Autodesk Inventor part; units mm, degrees
ref_plane "YZ Plane" through (0, 0, 0) normal (1, 0, 0) x (0, 1, 0)
ref_plane "XZ Plane" through (0, 0, 0) normal (0, 1, 0) x (-1, 0, 0)
ref_plane "XY Plane" through (0, 0, 0) normal (0, 0, 1) x (1, 0, 0)
sketch "Sketch1" plane through (0, 0, 0) normal (0, 0, 1) x (1, 0, 0)
  line L0 (0, 0) -> (44.45, 0)
  line L1 (44.45, 0) -> (44.45, 3.302)
  line L2 (44.45, 3.302) -> (3.302, 3.302)
  line L3 (0, 31.75) -> (0, 0)
  line L4 (3.302, 3.302) -> (3.302, 31.75)
  line L5 (3.302, 31.75) -> (0, 31.75)
  line L6 (0, 31.75) -> (0, 0)
  point P0 (0, 3.302)
  dimension "d1" = 3.302
  dimension "d2" = 3.302
  dimension "d50" = 44.45
  dimension "d57" = 31.75
extrude "Extrusion1" add sketch "Sketch1" along normal blind 50.8
sketch "Sketch3" plane through (0, 0, 0) normal (-1, 0, 0) x (0, 0, 1)
  line L0 (0, 0) -> (50.8, 0) construction
  line L1 (0, 0) -> (12.7, 0) construction
  line L2 (12.7, 0) -> (25.4, 0) construction
  line L3 (25.4, 0) -> (38.1, 0) construction
  line L4 (38.1, 0) -> (38.1, 12.7) construction
  line L5 (38.1, 12.7) -> (38.1, 25.4) construction
  line L6 (25.4, 0) -> (25.4, 12.7) construction
  line L7 (25.4, 12.7) -> (25.4, 25.4) construction
  line L8 (12.7, 0) -> (12.7, 12.7) construction
  line L9 (12.7, 12.7) -> (12.7, 25.4) construction
  circle A0 centre (12.7, 25.4) radius 2.5797
  circle A1 centre (25.4, 25.4) radius 2.5797
  circle A2 centre (38.1, 25.4) radius 2.5797
  circle A3 centre (38.1, 12.7) radius 2.5797
  circle A4 centre (25.4, 12.7) radius 2.5797
  circle A5 centre (12.7, 12.7) radius 2.5797
  dimension "d9" = 12.7
  dimension "d10" = 12.7
  dimension "d11" = 12.7
  dimension "d12" = 12.7
  dimension "d13" = 12.7
  dimension "d14" = 12.7
  dimension "d15" = 12.7
  dimension "d16" = 12.7
  dimension "d17" = 12.7
  dimension "d18" = 5.1594
  dimension "d19" = 5.1594
  dimension "d20" = 5.1594
  dimension "d21" = 5.1594
  dimension "d22" = 5.1594
  dimension "d23" = 5.1594
extrude "Extrusion3" cut sketch "Sketch3" against normal blind 50.8
sketch "Sketch4" plane through (0, 0, 0) normal (0, -1, 0) x (1, 0, 0)
  line L0 (44.45, 0) -> (44.45, 50.8) construction
  line L1 (44.45, 50.8) -> (44.45, 38.1) construction
  line L2 (50.8, 38.1) -> (44.45, 38.1) construction
  line L3 (44.45, 38.1) -> (31.75, 38.1) construction
  line L4 (31.75, 38.1) -> (19.05, 38.1) construction
  line L5 (44.45, 0) -> (44.45, 13.462) construction
  circle A0 centre (31.75, 38.1) radius 2.5797
  circle A1 centre (19.05, 38.1) radius 2.5797
  line L6 (50.8, 12.7) -> (44.45, 12.7) construction
  line L7 (44.45, 12.7) -> (31.75, 12.7) construction
  line L8 (31.75, 12.7) -> (19.05, 12.7) construction
  line L9 (19.05, 12.7) -> (6.35, 12.7) construction
  circle A2 centre (31.75, 12.7) radius 2.5797
  circle A3 centre (19.05, 12.7) radius 2.5797
  line L10 (44.45, 13.462) -> (38.1, 13.462) construction
  line L11 (44.45, 12.7) -> (44.45, 17.4414) construction
  line L12 (19.05, 38.1) -> (6.35, 38.1) construction
  point P0 (0, 0)
  dimension "d26" = 12.7
  dimension "d27" = 6.35
  dimension "d28" = 12.7
  dimension "d29" = 12.7
  dimension "d31" = 13.462
  dimension "d33" = 5.1594
  dimension "d34" = 5.1594
  dimension "d37" = 6.35
  dimension "d38" = 12.7
  dimension "d39" = 12.7
  dimension "d40" = 12.7
  dimension "d42" = 5.1594
  dimension "d43" = 5.1594
  dimension "d53" = 12.7
extrude "Extrusion7" cut sketch "Sketch4" against normal blind 25.4
properties part number "2in bracket"
The listing builds one solid part. Answer for the finished solid, in the listing's coordinates (mm). A direction names the side the tool comes from. Give positions to 0.01 mm unless a question says otherwise; leave off trailing zeros. Order: outer loops, then holes, each group sorted by start corner. A loop starts at its lowest first (then second) coordinate and runs counter-clockwise, first axis right, second up. Notation, with made-up numbers: M 1,71 L 51,71 A26 cw 51,91 Z; hole C 80.25,86 d8. An arc over 180 degrees is marked long. Put each result on its own line as item: value. Start each with the question number.
Item 1: The part is cut by section B-B, the plane z = 38.1. Determine the outline of the cut face in (x, y).
Item 2: The part is cut by section A-A, the plane y = 25.4. Determine the outline of the cut face in (x, z).
Item 3: Find the intervals of material crossed by line 1 along Y through (x, z) = (2.5, 12.7); line 2 along Z through (x, y) = (19, 1); line 3 along X through (y, z) = (1, 38), in increasing order.
Item 4: Which of the six approach directions +Z, -Z, +X, -X, +Y, -Y give full straight-line access (tool end or side, diameter ignored) to faces 5 (the face through (3.302, 17, 25)), 6 (the face through (44.45, 2, 25))?
Item 5: For a pull along Z with two mould halves and no side action, classify faces 1 (the face through (14, 3, 50.8)), 2 (the face through (24, 3.302, 25)), 3 (the face through (18.49, 1.63, 35.58)), 4 (the face through (1.628, 11.712, 15.083)) as +Z half, -Z half, draft (parallel to the pull), parting line (faces both ways), or undercut.
Item 6: Flat-ended cylindrical pins translate along their axes: P1, Ø8.5, axis at y = 12.7, z = 25.4, coming from the -X side; P2, Ø6.5, axis at y = 25.4, z = 25.4, coming from the +X side. Find the tip coordinate at first contact, or state that the pin passes through.
Item 7: The part is cut by section C-C, the plane x = 19.05. Determine the outline of the cut face in (y, z).
Item 8: The part is cut by section D-D, the plane z = 9. Determine the outline of the cut face in (x, y), and give its area (3 significant figures).
Answer key:
1. outline: M 0,0 L 16.47,0 L 16.47,3.3 L 3.3,3.3 L 3.3,10.12 L 0,10.12 Z; M 0,15.28 L 3.3,15.28 L 3.3,22.82 L 0,22.82 Z; M 0,27.98 L 3.3,27.98 L 3.3,31.75 L 0,31.75 Z; M 21.63,0 L 29.17,0 L 29.17,3.3 L 21.63,3.3 Z; M 34.33,0 L 44.45,0 L 44.45,3.3 L 34.33,3.3 Z
2. outline: M 0,0 L 3.3,0 L 3.3,10.12 L 0,10.12 Z; M 0,15.28 L 3.3,15.28 L 3.3,22.82 L 0,22.82 Z; M 0,27.98 L 3.3,27.98 L 3.3,35.52 L 0,35.52 Z; M 0,40.68 L 3.3,40.68 L 3.3,50.8 L 0,50.8 Z
3. line 1: y = 0 to 10.12, 15.28 to 22.82, 27.98 to 31.75
3. line 2: z = 0 to 10.12, 15.28 to 35.52, 40.68 to 50.8
3. line 3: x = 0 to 16.47, 21.63 to 29.17, 34.33 to 44.45
4. face 5: +Z, -Z, +X, +Y
4. face 6: +Z, -Z, +X, +Y, -Y
5. face 1: +Z half
5. face 2: draft
5. face 3: undercut
5. face 4: undercut
6. P1: stops at x = 0
6. P2: stops at x = 3.3
7. outline: M 0,0 L 3.3,0 L 3.3,10.12 L 0,10.12 Z; M 0,15.28 L 3.3,15.28 L 3.3,35.52 L 0,35.52 Z; M 0,40.68 L 3.3,40.68 L 3.3,50.8 L 0,50.8 Z
8. outline: M 0,0 L 44.45,0 L 44.45,3.3 L 3.3,3.3 L 3.3,31.75 L 0,31.75 Z
8. area: 241 mm²
